Work out the finished part from the listing and answer in its coordinate system (mm). Coordinates: 2 decimals unless noted, no trailing zeros. Order: outer loops, then holes, each group sorted by start corner. A loop starts at its lowest first (then second) coordinate and runs counter-clockwise, first axis right, second up. Notation, with made-up numbers: M 59,71 L 95,71 A25 ccw 95,108 Z; hole C 49.25,-22 d4. An arc over 180 degrees is marked long. Answer in a Markdown table with one row per item. Add a question column.
Item 1: The part is cut by section D-D (z = -54.8). Write down the section's boundary in (x, y), then the cut area to 3 significant figures.
Item 2: The part is cut by section A-A (z = -56.7). Write down the section's boundary in (x, y), then the cut area to 3 significant figures.
Item 3: The part is cut by section C-C (y = 30). Write down the section's boundary in (x, z).
Item 4: A flat-ended cylindrical pin translates along its axis: pin 1 Ø1.5 at (x, z) = (7, -55.5) entering from -Y. Find the tip coordinate at first contact, or state that the pin passes through.
Item 5: Consider line 1 (X direction, y = 25.25, z = -56.85); line 2 (Y direction, x = -6.5, z = -54.9); line 3 (X direction, y = 29, z = -55.2). Determine where each line is inside the solid, lowest interval first. Write a range as from..to.
Item 6: The part is cut by section B-B (x = 0). Write down the section's boundary in (y, z), then the cut area to 3 significant figures.
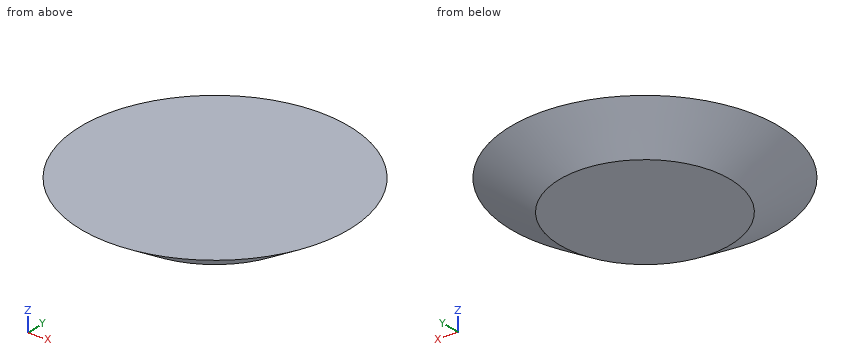
from build123d import *


with BuildPart() as obj1:
    # Cone → Cone (revolve)
    with BuildSketch(Plane(origin=(0, -30, 57), x_dir=(1, 0, 0), z_dir=(0, 1, 0))):
        Polygon((0, 0), (7, 0), (11, 2.5), (0, 2.5), align=None)
    revolve(axis=Axis((0, -30, 57), (0, 0, -1)))


with BuildPart() as obj2:
    # Part__Mirroring001: instance of obj1
    add(obj1.part.mirror(Plane(origin=(0, 0, 0), x_dir=(1, 0, 0), z_dir=(0, 1, 0))))


with BuildPart() as obj3:
    # Part__Mirroring005: instance of obj2
    add(obj2.part.mirror(Plane(origin=(0, 0, 0), x_dir=(0, 1, 0), z_dir=(0, 0, 1))))


solid = obj3.part
Reply:
| question | item | result |
|---|---|---|
| 1 | outline | C 0,30 d21.04 |
| 1 | area | 348 mm2 |
| 2 | outline | C 0,30 d14.96 |
| 2 | area | 176 mm2 |
| 3 | outline | M -11,-54.5 L -7,-57 L 7,-57 L 11,-54.5 Z |
| 4 | pin 1 | stops at y = 21.91 |
| 5 | line 1 | x = -5.46..5.46 |
| 5 | line 2 | y = 21.93..38.07 |
| 5 | line 3 | x = -9.83..9.83 |
| 6 | outline | M 19,-54.5 L 23,-57 L 37,-57 L 41,-54.5 Z |
| 6 | area | 45.0 mm2 |
